```python
from build123d import *

# Parameters (mm, degrees)
F0_W        = 126.7489343882
F0_H        = 41.312854737
F1_DEPTH    = 25.4
F2_R        = 22.987
F3_DEPTH    = 41.313854737
F4_T1_DEPTH = 76.2
F4_T3_DEPTH = 152.1489343882
F5_T1_DEPTH = 152.1484343931
F5_T3_DEPTH = 76.1995000049
F6_W        = 67.343034428
F6_H        = 15.8471396435
F7_DEPTH    = 41.313854837


# Not quite as in the source:
# - a fillet or chamfer that OpenCascade refuses, or shapes differently, is made with other operations: its cross-section is extruded or revolved along the edge and cut away or added


with BuildPart() as f1:
    # F0 (on Top) → F1 (new body, symmetric)
    with BuildSketch(Plane.XY):
        Rectangle(F0_W, F0_H)
    extrude(amount=F1_DEPTH, both=True)

    # F2 (on face) → F3 (cut, through all)
    with BuildSketch(Plane.XZ.offset(20.6564273685)):
        with Locations((-36.7568694055, 0)):
            Circle(F2_R)
    extrude(amount=-F3_DEPTH, mode=Mode.SUBTRACT)

    # F4: fillet of radius 5.08 on 5 edges, made by hand

    # F4_s2 → F4_t1 (cut)
    with BuildSketch(Plane.XY.offset(-38.1)):
        with BuildLine():
            ThreePointArc((-63.3744671941, -15.5764273685), (-61.8865696425, -19.1685298169), (-58.2944671941, -20.6564273685))
            Line((-58.2944671941, -20.6564273685), (-63.3744671941, -20.6564273685))
            Line((-63.3744671941, -20.6564273685), (-63.3744671941, -15.5764273685))
        make_face()
        with BuildLine():
            ThreePointArc((63.3744671941, -15.5764273685), (61.8865696425, -19.1685298169), (58.2944671941, -20.6564273685))
            Line((58.2944671941, -20.6564273685), (63.3744671941, -20.6564273685))
            Line((63.3744671941, -20.6564273685), (63.3744671941, -15.5764273685))
        make_face()
    extrude(amount=F4_T1_DEPTH, mode=Mode.SUBTRACT)

    # F4_s4 → F4_t3 (cut)
    with BuildSketch(Plane.YZ.offset(-76.0744671941)):
        with BuildLine():
            ThreePointArc((-15.5764273685, -25.4), (-19.1685298169, -23.9121024484), (-20.6564273685, -20.32))
            Line((-20.6564273685, -20.32), (-20.6564273685, -25.4))
            Line((-20.6564273685, -25.4), (-15.5764273685, -25.4))
        make_face()
        with BuildLine():
            ThreePointArc((-15.5764273685, 25.4), (-19.1685298169, 23.9121024484), (-20.6564273685, 20.32))
            Line((-20.6564273685, 20.32), (-20.6564273685, 25.4))
            Line((-20.6564273685, 25.4), (-15.5764273685, 25.4))
        make_face()
    extrude(amount=F4_T3_DEPTH, mode=Mode.SUBTRACT)

    # F4_s5 → F4_t6 (revolve, cut)
    with BuildSketch(Plane.XY):
        with BuildLine():
            ThreePointArc((-13.7698694055, -15.5764273685), (-12.2819718539, -19.1685298169), (-8.6898694055, -20.6564273685))
            Line((-8.6898694055, -20.6564273685), (-13.7698694055, -20.6564273685))
            Line((-13.7698694055, -20.6564273685), (-13.7698694055, -15.5764273685))
        make_face()
    revolve(axis=Axis((-36.7568694055, -20.6564273685, 0), (0, -1, 0)), mode=Mode.SUBTRACT)

    # F5: fillet of radius 5.08 on 5 edges, made by hand

    # F5_s2 → F5_t1 (cut)
    with BuildSketch(Plane.YZ.offset(-76.0742171965)):
        with BuildLine():
            ThreePointArc((20.6565273685, -20.3201), (19.1686298169, -23.9122024484), (15.5765273685, -25.4001))
            Line((15.5765273685, -25.4001), (15.5765273685, -25.5017))
            ThreePointArc((15.5765273685, -25.5017), (18.1164773685, -25.5016), (20.6564273685, -25.5016))
            Line((20.6564273685, -25.5016), (20.7580273685, -25.4))
            ThreePointArc((20.7580273685, -25.4), (20.7580273685, -22.86005), (20.7581273685, -20.3201))
            Line((20.7581273685, -20.3201), (20.6565273685, -20.3201))
        make_face()
        with BuildLine():
            ThreePointArc((20.6565273685, 20.3201), (19.1686298169, 23.9122024484), (15.5765273685, 25.4001))
            Line((15.5765273685, 25.4001), (15.5765273685, 25.5017))
            ThreePointArc((15.5765273685, 25.5017), (18.1164773685, 25.5016), (20.6564273685, 25.5016))
            Line((20.6564273685, 25.5016), (20.7580273685, 25.4))
            ThreePointArc((20.7580273685, 25.4), (20.7580273685, 22.86005), (20.7581273685, 20.3201))
            Line((20.7581273685, 20.3201), (20.6565273685, 20.3201))
        make_face()
    extrude(amount=F5_T1_DEPTH, mode=Mode.SUBTRACT)

    # F5_s4 → F5_t3 (cut)
    with BuildSketch(Plane.XY.offset(-38.0997500025)):
        with BuildLine():
            ThreePointArc((58.2945671941, 20.6565273685), (61.8866696425, 19.1686298169), (63.3745671941, 15.5765273685))
            Line((63.3745671941, 15.5765273685), (63.4761671941, 15.5765273685))
            ThreePointArc((63.4761671941, 15.5765273685), (63.4760671941, 18.1164773685), (63.4760671941, 20.6564273685))
            Line((63.4760671941, 20.6564273685), (63.3744671941, 20.7580273685))
            ThreePointArc((63.3744671941, 20.7580273685), (60.8345171941, 20.7580273685), (58.2945671941, 20.7581273685))
            Line((58.2945671941, 20.7581273685), (58.2945671941, 20.6565273685))
        make_face()
        with BuildLine():
            ThreePointArc((-58.2945671941, 20.6565273685), (-61.8866696425, 19.1686298169), (-63.3745671941, 15.5765273685))
            Line((-63.3745671941, 15.5765273685), (-63.4761671941, 15.5765273685))
            ThreePointArc((-63.4761671941, 15.5765273685), (-63.4760671941, 18.1164773685), (-63.4760671941, 20.6564273685))
            Line((-63.4760671941, 20.6564273685), (-63.3744671941, 20.7580273685))
            ThreePointArc((-63.3744671941, 20.7580273685), (-60.8345171941, 20.7580273685), (-58.2945671941, 20.7581273685))
            Line((-58.2945671941, 20.7581273685), (-58.2945671941, 20.6565273685))
        make_face()
    extrude(amount=F5_T3_DEPTH, mode=Mode.SUBTRACT)

    # F5_s5 → F5_t6 (revolve, cut)
    with BuildSketch(Plane.XY):
        with BuildLine():
            ThreePointArc((-8.6899694055, 20.6565273685), (-12.2820718539, 19.1686298169), (-13.7699694055, 15.5765273685))
            Line((-13.7699694055, 15.5765273685), (-13.8715694055, 15.5765273685))
            ThreePointArc((-13.8715694055, 15.5765273685), (-13.8714694055, 18.1164773685), (-13.8714694055, 20.6564273685))
            Line((-13.8714694055, 20.6564273685), (-13.7698694055, 20.7580273685))
            ThreePointArc((-13.7698694055, 20.7580273685), (-11.2299194055, 20.7580273685), (-8.6899694055, 20.7581273685))
            Line((-8.6899694055, 20.7581273685), (-8.6899694055, 20.6565273685))
        make_face()
    revolve(axis=Axis((-36.7568694055, 20.6564273685, 0), (0, -1, 0)), mode=Mode.SUBTRACT)

    # F6 (on face) → F7 (cut, through all)
    with BuildSketch(Plane(origin=(0, 20.6564273685, 0), x_dir=(-1, 0, 0), z_dir=(0, 1, 0))):
        with Locations((-24.6229499801, -12.3964301783)):
            Rectangle(F6_W, F6_H)
        with Locations((-24.6229499801, 12.3964301783)):
            Rectangle(F6_W, F6_H)
    extrude(amount=-F7_DEPTH, mode=Mode.SUBTRACT)


solid = f1.part
```
Read the model definition and answer for the solid it produces. Units are mm, in the model's axes. A direction names the side the tool comes from. Round coordinates to 2 decimals unless told otherwise and drop trailing zeros. Loops run counter-clockwise (first coordinate to the right, second up) from the corner with the lowest first, then second, coordinate; pieces in that order, holes last. Notation, with made-up numbers: (-40, 8.5) -> (-8, 8.5) arc R13 ccw to (-8, 16.5) -> close; hole circle Ø8 at (36, 20). An arc over 180 degrees is marked (long way). One line per item, written item: value.
1) A cutting plane is placed at B-B (y = -7). Determine the outline of the cut face in (x, z).
Answer list:
outline: (-63.37, -25.4) -> (63.37, -25.4) -> (63.37, 25.4) -> (-63.37, 25.4) -> close; hole circle Ø45.97 at (-36.76, 0); hole (-9.05, -20.32) -> (58.29, -20.32) -> (58.29, -4.47) -> (-9.05, -4.47) -> close; hole (-9.05, 4.47) -> (58.29, 4.47) -> (58.29, 20.32) -> (-9.05, 20.32) -> close
2) A flat-ended cylindrical pin translates along its axis: P1, Ø12, axis at x = -19.5, z = -8.5, coming from the -Y side. Find the tip coordinate at first contact, or state that the pin passes through.
Answer list:
P1: stops at y = -19.79
3) Consider L1, parallel to Z at x = 43, y = -6; L2, parallel to X at y = -9, z = 0; L3, parallel to X at y = 10, z = 8.5. Determine where each line is inside the solid, lowest interval first. Write a range as [from, to].
Answer list:
L1: z = [-25.4, -20.32], [-4.47, 4.47], [20.32, 25.4]
L2: x = [-63.37, -59.74], [-13.77, 63.37]
L3: x = [-63.37, -58.11], [-15.4, -9.05], [58.29, 63.37]
4) A cutting plane is placed at A-A (x = 1.5). Give the number of separate pieces and of enclosed holes in the cut face, and give its area (3 significant figures).
Answer list:
separate pieces: 3
enclosed holes: 0
area: 767 mm²
5) For faces 5 (the face through (25, 0, -4.473)), 6 (the face through (-58, -20.656, 20)), determine the directions among +Z, -Z, +X, -X, +Y, -Y from which every point of the face is accessible in a straight line to the end or side of a thin tool.
Answer list:
face 5: +Y, -Y
face 6: +Z, -Z, +X, -X, -Y
6) A cutting plane is placed at C-C (z = 0). Determine the outline of the cut face in (x, y).
Answer list:
outline: (-63.37, -15.58) arc R5.08 ccw to (-61.56, -19.47) arc R5.08 ccw to (-59.74, -15.58) -> (-59.74, 15.61) arc R5.08 ccw to (-61.56, 19.47) arc R5.08 ccw to (-63.37, 15.61) -> close; (-13.77, -15.58) arc R5.08 ccw to (-8.69, -20.66) -> (58.29, -20.66) arc R5.08 ccw to (63.37, -15.58) -> (63.37, 15.61) arc R5.08 ccw to (58.33, 20.66) -> (-8.72, 20.66) arc R5.08 ccw to (-13.77, 15.61) -> close
7) The mould has two halves that part along X. Classify faces 1 (the face through (61.847, 19.208, -0.356)), 2 (the face through (-1, 0, -25.4)), 3 (the face through (25, 0, -20.32)), 4 (the face through (58.294, 0, 12)): pulls with the +X half, pulls with the -X half, needs draft (parallel to the pull), parting line crosses it, or undercut.
Answer list:
face 1: pulls with the +X half
face 2: needs draft
face 3: undercut
face 4: undercut
